```python
from build123d import *

# Parameters (mm, degrees)
SKETCH_1_W          = 80
SKETCH_1_H          = 30
SKETCH_1_R          = 9
EXTRUDE_1_DEPTH     = 5
EXTRUDE_START       = 1.5
SKETCH_4_R          = 11
SKETCH_4_R_2        = 9
EXTRUDE_4_DEPTH     = 1.5
SKETCH_5_R          = 32
SKETCH_5_R_2        = 26
CUT_EXTRUDE_1_DEPTH = 3
SKETCH_8_R          = 1.5
CUT_EXTRUDE_2_DEPTH = 10
FILLET_1_R          = 3
CHAMFER_1_SIZE      = 0.5


with BuildPart() as part:
    # 草图1 → 凸台-拉伸1 (new body)
    with BuildSketch(Plane(origin=(0, 0, 0), x_dir=(1, 0, 0), z_dir=(0, 1, 0))):
        Rectangle(SKETCH_1_W, SKETCH_1_H)
        with Locations(Location((0, 0, 0), (0, 0, 270))):
            Circle(SKETCH_1_R, mode=Mode.SUBTRACT)
    extrude(amount=-EXTRUDE_1_DEPTH)

    # 草图4 → 凸台-拉伸4 (add)
    with BuildSketch(Plane(origin=(0, 0, 0), x_dir=(1, 0, 0), z_dir=(0, 1, 0)).offset(EXTRUDE_START)):
        with Locations(Location((0, 0, 0), (0, 0, 270))):
            Circle(SKETCH_4_R)
        with Locations(Location((0, 0, 0), (0, 0, 270))):
            Circle(SKETCH_4_R_2, mode=Mode.SUBTRACT)
    extrude(amount=-EXTRUDE_4_DEPTH)

    # 草图5 → 切除-拉伸1 (cut)
    with BuildSketch(Plane(origin=(0, 0, 0), x_dir=(1, 0, 0), z_dir=(0, 1, 0))):
        Circle(SKETCH_5_R)
        Circle(SKETCH_5_R_2, mode=Mode.SUBTRACT)
    extrude(amount=-CUT_EXTRUDE_1_DEPTH, mode=Mode.SUBTRACT)

    # 草图8 → 切除-拉伸2 (cut)
    with BuildSketch(Plane.XZ.offset(5)):
        with Locations(Location((35, 10, 0), (0, 0, 270))):
            Circle(SKETCH_8_R)
        with Locations(Location((35, -10, 0), (0, 0, 270))):
            Circle(SKETCH_8_R)
        with Locations(Location((-35, -10, 0), (0, 0, 90))):
            Circle(SKETCH_8_R)
        with Locations(Location((-35, 10, 0), (0, 0, 90))):
            Circle(SKETCH_8_R)
    extrude(amount=-CUT_EXTRUDE_2_DEPTH, mode=Mode.SUBTRACT)

    # 圆角1
    fillet_1_edges = [part.edges().sort_by_distance(p)[0] for p in [
        (28.26658805, -1.5, 15),
        (-28.26658805, -1.5, 15),
        (-28.26658805, -1.5, -15),
        (28.26658805, -1.5, -15),
        (21.236760582, -1.5, 15),
        (21.236760582, -1.5, -15),
        (-21.236760582, -1.5, 15),
        (-21.236760582, -1.5, -15),
        (40, -2.5, 15),
        (-40, -2.5, 15),
        (-40, -2.5, -15),
        (40, -2.5, -15),
    ]]
    fillet(fillet_1_edges, radius=FILLET_1_R)

    # 倒角1
    chamfer_1_edges = [part.edges().sort_by_distance(p)[0] for p in [
        (0, 1.5, -11),
    ]]
    chamfer(chamfer_1_edges, length=CHAMFER_1_SIZE)


solid = part.part
```
Verification items for the finished model (mm, model axes). A direction names the side the tool comes from. Coordinates: 2 decimals unless noted, no trailing zeros. Loops run counter-clockwise (first coordinate to the right, second up) from the corner with the lowest first, then second, coordinate; pieces in that order, holes last. Notation, with made-up numbers: (-8, 59) - (20, 59) arc R36 cw to (20, 98) - close; hole circle Ø9 at (39.5, 38.25). An arc over 180 degrees is marked (long way). Answer as a JSON object with one key per item and string values.
(1) Mould release check, pull along X, two halves, no side actions. Record for faces 4 (the flat face through (40, -2, 0)), 5 (the cylindrical face through (-30.44, -1.48, 13.75)), 6 (the flat face through (-35, 0, 0)), 7 (the cylindrical face through (21.107, -1.479, -14.606)): pulls with the +X half, pulls with the -X half, needs draft (parallel to the pull), parting line crosses it, or undercut.
Response:
{"face 4": "pulls with the +X half", "face 5": "undercut", "face 6": "needs draft", "face 7": "undercut"}
(2) Scan lines: line 1 along Z through (x, y) = (-35, -3.4); line 2 along Z through (x, y) = (3, -4.5); line 3 along X through (y, z) = (-3.4, 10). Record each from-to range of solid material in increasing order.
Response:
{"line 1": "z = -15 to -11.5, -8.5 to 8.5, 11.5 to 15", "line 2": "z = -15 to -8.49, 8.49 to 15", "line 3": "x = -40 to -36.5, -33.5 to 33.5, 36.5 to 40"}
(3) Cross-section at B-B, the plane x = -35. Record the boundary of the cut face in (y, z), then the cut area to 3 significant figures.
Response:
{"outline": "(-5, -15) - (0, -15) - (0, -11.5) - (-5, -11.5) - close; (-5, -8.5) - (0, -8.5) - (0, 8.5) - (-5, 8.5) - close; (-5, 11.5) - (0, 11.5) - (0, 15) - (-5, 15) - close", "area": "120 mm²"}
(4) Access from +Z, -Z, +X, -X, +Y, -Y to the whole of each face (thin tool, end or side, straight path). Record for faces 1 (the cylindrical face through (26, -1, 0)), 2 (the cylindrical face through (-39.1, -2.54, -14.14)), 3 (the flat face through (36, 0, 0)).
Response:
{"face 1": "+Y", "face 2": "-Z, -X, +Y, -Y", "face 3": "+Z, -Z, +X, +Y"}
(5) Cross-section at A-A, the plane y = -2. Count the separate pieces of the cut face and the enclosed holes in it, then the cut area to 3 significant figures.
Response:
{"separate pieces": "3", "enclosed holes": "5", "area": "1,710 mm²"}
(6) Go/stop test with a flat-tipped pin: pin 1 Ø3 at (x, z) = (-34.5, -7) entering from +Y. Record where the tip stops, or that it passes through.
Response:
{"pin 1": "stops at y = 0"}
